from build123d import *

# Parameters (mm, degrees)
F0_W     = 203.2
F0_H     = 508
F0_W_2   = 50.8
F0_H_2   = 152.4
F0_H_3   = 203.2
F1_DEPTH = 50.8


with BuildPart() as f1:
    # F0 (on Front) → F1 (new body)
    with BuildSketch(Plane.XZ):
        with Locations((-990.6, -838.2)):
            Rectangle(F0_W, F0_H)
        with Locations((-990.6, -812.8)):
            Rectangle(F0_W_2, F0_H_2, mode=Mode.SUBTRACT)
        with Locations((990.6, -838.2)):
            Rectangle(F0_W, F0_H)
        with Locations((990.6, -812.8)):
            Rectangle(F0_W_2, F0_H_2, mode=Mode.SUBTRACT)
        with BuildLine():
            add(Edge.make_bspline(
                [(-1092.2, 584.2), (-980.9341244819, 539.9121567226), (-692.3205033902, 468.9691085106), (-103.7885392301, 611.398573737), (693.6453585688, 466.7257971096), (995.3503534145, 539.0780902978), (1092.2, 584.2)],
                knots=[0, 0, 0, 0, 0.2126532774, 0.4794774151, 0.7873467226, 1, 1, 1, 1], degree=3))
            Line((-1092.2, 584.2), (-1092.2, -584.2))
            Line((-1092.2, -584.2), (-889, -584.2))
            Line((-889, -584.2), (889, -584.2))
            Line((889, -584.2), (1092.2, -584.2))
            Line((1092.2, -584.2), (1092.2, 584.2))
        make_face()
        with Locations((-596.9, 228.6)):
            Rectangle(F0_W, F0_H_3, mode=Mode.SUBTRACT)
        with Locations((0, 228.6)):
            Rectangle(F0_W, F0_H_3, mode=Mode.SUBTRACT)
        with Locations((596.9, 228.6)):
            Rectangle(F0_W, F0_H_3, mode=Mode.SUBTRACT)
    extrude(amount=F1_DEPTH)


solid = f1.part
Can you work these out from the model? Positions are in its coordinate system, mm. A direction names the side the tool comes from. Coordinates: 2 decimals unless noted, no trailing zeros. Loops run counter-clockwise (first coordinate to the right, second up) from the corner with the lowest first, then second, coordinate; pieces in that order, holes last. Notation, with made-up numbers: M 85.5,-8 L 137.5,-8 A28 ccw 137.5,17 Z; hole C 26.25,-5.5 d5. An arc over 180 degrees is marked long. Return JSON: item names as keys, results as strings. Group by question number.
Item 1: Imagine slicing it at B-B (y = -30). Give the number of separate pieces and of enclosed holes in the cut face, and give its area (3 significant figures).
Item 2: If I drill on L1, parallel to X at y = -3, z = 254; L2, parallel to X at y = -18.5, z = -763.5; L3, parallel to X at y = -29, z = -994.5, over which ranges is the centre line in solid material (lowest first)? Write a range as from..to.
Item 3: Imagine slicing it at A-A (z = 261.5). Please give me the cut outline in (x, y), and give its area (3 significant figures).
Item 4: Thinking about a two-plate mould opening in X: for faces 4 (the flat face through (1092.2, -25, -266)), 5 (the flat face through (990, -25, -736.6)), 6 (the flat face through (-101.6, -25, 227)), 7 (the flat face through (-15, -50.8, -39)), which applies, released by +X, released by -X, zero draft, split by the parting line, or undercut?
Item 5: I'm going to push flat-ended pins straight in: pin 1 Ø8 at (x, y) = (850.5, -40) entering from +Z; pin 2 Ø3 at (x, y) = (766.5, -35) entering from +Z; pin 3 Ø15 at (x, y) = (-988, -25.5) entering from +Z. Where does each tip first touch, or does it pass through?
Item 6: On a 3-axis mill with a long thin cutter (end or side, diameter ignored), from which of +Z, -Z, +X, -X, +Y, -Y can I reach the whole of each face in a straight line? I mean faces 1 (the flat face through (889, -25, -842)), 2 (the flat face through (101.6, -25, 227)), 3 (the flat face through (989, -25, -1092.2)). Say none if no direction works.
Verdict:
{
 "1": {"separate pieces": "1", "enclosed holes": "5", "area": "2,510,000 mm^2"},
 "2": {"L1": "x = -1092.2..-698.5, -495.3..-101.6, 101.6..495.3, 698.5..1092.2", "L2": "x = -1092.2..-1016, -965.2..-889, 889..965.2, 1016..1092.2", "L3": "x = -1092.2..-889, 889..1092.2"},
 "3": {"outline": "M -1092.2,-50.8 L -698.5,-50.8 L -698.5,0 L -1092.2,0 Z; M -495.3,-50.8 L -101.6,-50.8 L -101.6,0 L -495.3,0 Z; M 101.6,-50.8 L 495.3,-50.8 L 495.3,0 L 101.6,0 Z; M 698.5,-50.8 L 1092.2,-50.8 L 1092.2,0 L 698.5,0 Z", "area": "80,000 mm^2"},
 "4": {"face 4": "released by +X", "face 5": "undercut", "face 6": "undercut", "face 7": "zero draft"},
 "5": {"pin 1": "stops at z = 517.67", "pin 2": "stops at z = 509.76", "pin 3": "stops at z = 550.6"},
 "6": {"face 1": "-Z, +Y, -Y", "face 2": "+Y, -Y", "face 3": "-Z, +X, -X, +Y, -Y"}
}
